Source: CAD feature listing. Evaluate the final solid. Frame: model axes, mm. A direction names the side the tool comes from. Round coordinates to 2 decimals unless told otherwise and drop trailing zeros. Write each loop counter-clockwise with the first axis right and the second up, starting at its lowest first coordinate (ties: lowest second). Pieces come first, ordered by that corner, then holes. Notation, with made-up numbers: M -2.5,50.5 L 38.5,50.5 A37 ccw 38.5,88.5 Z; hole C -15.75,47 d9. An arc over 180 degrees is marked long. Answer in a Markdown table with one row per item.
from build123d import *

# Parameters (mm, degrees)
SKETCH2_R           = 17.6
BOSS_EXTRUDE1_DEPTH = 52.5
SKETCH3_R           = 2.1
BOSS_EXTRUDE2_DEPTH = 7.6
SKETCH4_W           = 1.23
SKETCH4_H           = 14.7
BOSS_EXTRUDE3_DEPTH = 3.5
CUT_EXTRUDE1_START  = -3
SKETCH5_R           = 17.6
SKETCH5_R_2         = 4.5
SKETCH5_W           = 1.23
SKETCH5_H           = 14.7
SKETCH5_R_3         = 2.5
CUT_EXTRUDE1_DEPTH  = 3
SKETCH7_R           = 19.95
BOSS_EXTRUDE5_DEPTH = 5.5
FILLET3_R           = 5
FILLET4_R           = 0.5
CUT_EXTRUDE2_START  = -7
SKETCH8_R           = 2.5
CUT_EXTRUDE2_DEPTH  = 7
SKETCH10_R          = 2.8
BOSS_EXTRUDE6_DEPTH = 8.6
FILLET5_R           = 0.5


with BuildPart() as part:
    # Sketch2 → Boss-Extrude1 (new body)
    with BuildSketch(Plane.XY):
        Circle(SKETCH2_R)
    extrude(amount=BOSS_EXTRUDE1_DEPTH)

    # Sketch3 → Boss-Extrude2 (add)
    # profile 1 of 2: a face of its own
    with BuildSketch(Plane.XY):
        with BuildLine():
            Line((-10.476190476, 14.14246913), (-25.391666667, 3.093665122))
            ThreePointArc((-25.391666667, 3.093665122), (-26.95, 0), (-25.391666667, -3.093665122))
            Line((-25.391666667, -3.093665122), (-10.476190476, -14.14246913))
            ThreePointArc((-10.476190476, -14.14246913), (-17.6, 0), (-10.476190476, 14.14246913))
        make_face()
        with Locations(Location((-23.1, 0, 0), (0, 0, 180))):
            Circle(SKETCH3_R, mode=Mode.SUBTRACT)
    # profile 2 of 2: a face of its own
    with BuildSketch(Plane.XY):
        with BuildLine():
            Line((25.391666667, 3.093665122), (10.476190476, 14.14246913))
            ThreePointArc((10.476190476, 14.14246913), (17.6, 0), (10.476190476, -14.14246913))
            Line((10.476190476, -14.14246913), (25.391666667, -3.093665122))
            ThreePointArc((25.391666667, -3.093665122), (26.95, 0), (25.391666667, 3.093665122))
        make_face()
        with Locations(Location((23.1, 0, 0), (0, 0, 180))):
            Circle(SKETCH3_R, mode=Mode.SUBTRACT)
    extrude(amount=BOSS_EXTRUDE2_DEPTH)

    # Sketch4 → Boss-Extrude3 (add)
    with BuildSketch(Plane.XY.offset(52.5)):
        Rectangle(SKETCH4_W, SKETCH4_H)
    extrude(amount=BOSS_EXTRUDE3_DEPTH)

    # Sketch5 → Cut-Extrude1 (cut)
    # profile 1 of 3: a face of its own
    with BuildSketch(Plane.XY.offset(52.5).offset(CUT_EXTRUDE1_START)):
        with Locations(Location((0, 0, 0), (0, 0, 126.52960723))):
            Circle(SKETCH5_R)
        with Locations((-8.9, 0)):
            Circle(SKETCH5_R_2, mode=Mode.SUBTRACT)
        with Locations((8.9, 0)):
            Circle(SKETCH5_R_2, mode=Mode.SUBTRACT)
        Rectangle(SKETCH5_W, SKETCH5_H, mode=Mode.SUBTRACT)
    # profile 2 of 3: a face of its own
    with BuildSketch(Plane.XY.offset(52.5).offset(CUT_EXTRUDE1_START)):
        with Locations((-8.9, 0)):
            Circle(SKETCH5_R_3)
    # profile 3 of 3: a face of its own
    with BuildSketch(Plane.XY.offset(52.5).offset(CUT_EXTRUDE1_START)):
        with Locations((8.9, 0)):
            Circle(SKETCH5_R_3)
    extrude(amount=CUT_EXTRUDE1_DEPTH, mode=Mode.SUBTRACT)

    # Sketch7 → Boss-Extrude5 (add)
    with BuildSketch(Plane.XY.offset(49.5)):
        Circle(SKETCH7_R)
    extrude(amount=-BOSS_EXTRUDE5_DEPTH)

    # Fillet3
    # the kernel refuses this fillet: 5 mm, written as the material it adds along each edge
    with BuildSketch(Plane(origin=(0, 0, 44), x_dir=(1, 0, 0), z_dir=(0, 1, 0))) as fillet3_piece_1:
        with BuildLine():
            CenterArc((22.6, 4.239988208), FILLET3_R, 180, 57.994545172)
            Line((19.95, 0), (19.897, -0.084799764))
            ThreePointArc((19.897, -0.084799764), (18.775, -0.1), (17.6, -0.1))
            Line((17.6, -0.1), (17.5, 0))
            Line((17.5, 0), (17.5, 4.239988208))
            Line((17.5, 4.239988208), (17.6, 4.239988208))
        make_face()
    revolve(axis=Axis((0, 0, 44), (0, 0, -1)))

    # Fillet4
    fillet4_edges = [part.edges().sort_by_distance(p)[0] for p in [
        (0.615, 0, 56),
        (0, 7.35, 56),
        (0, -7.35, 56),
        (-0.615, 0, 56),
        (0, 7.35, 49.5),
        (-0.615, 0, 49.5),
        (0, -7.35, 49.5),
        (0.615, 0, 49.5),
        (-13.4, 0, 49.5),
        (4.4, 0, 49.5),
        (-19.95, 0, 49.5),
    ]]
    fillet(fillet4_edges, radius=FILLET4_R)

    # Sketch8 → Cut-Extrude2 (cut)
    with BuildSketch(Plane.XY.offset(52.5).offset(CUT_EXTRUDE2_START)):
        with Locations((8.9, 0)):
            Circle(SKETCH8_R)
        with Locations((-8.9, 0)):
            Circle(SKETCH8_R)
    extrude(amount=CUT_EXTRUDE2_DEPTH, mode=Mode.SUBTRACT)

    # Sketch10 → Boss-Extrude6 (add)
    with BuildSketch(Plane.XY.offset(49.5)):
        with Locations(Location((0, 12.15, 0), (0, 0, 180))):
            Circle(SKETCH10_R)
    extrude(amount=BOSS_EXTRUDE6_DEPTH)

    # Fillet5
    fillet5_edges = [part.edges().sort_by_distance(p)[0] for p in [
        (2.8, 12.15, 58.1),
    ]]
    fillet(fillet5_edges, radius=FILLET5_R)


solid = part.part
Q1. Contact query for flat-ended pins moving along their axis: pin 1 Ø4 at (x, z) = (15, 16.5) entering from +Y; pin 2 Ø4.5 at (y, z) = (-2, 51.5) entering from -X; pin 3 Ø1 at (x, z) = (-14, 21) entering from -Y. Output: stop coordinate, or through.
Solutions:
| item | result |
|---|---|
| pin 1 | stops at y = 11.86 |
| pin 2 | stops at x = -19.8 |
| pin 3 | stops at y = -11.29 |
Q2. Material intervals for probe 1 along X at (y, z) = (0.5, 51) (3 decimals); probe 2 along Y at (x, z) = (-8.9, 51); probe 3 along Z at (x, y) = (-12, -6), sorted ascending.
Solutions:
| item | result |
|---|---|
| probe 1 | x = -13.372 to -11.349, -6.451 to -4.428, -0.615 to 0.615, 4.428 to 6.451, 11.349 to 13.372 |
| probe 2 | y = -4.5 to -2.5, 2.5 to 4.5 |
| probe 3 | z = 0 to 49.5 |
Q3. Access query for faces 4 (the flat face through (-7, -2, 52.5)), 5 (the flat face through (17.83, -8.695, 3.747)), 6 (the flat face through (4, -4, 49.5)), 7 (the flat face through (11, -2, 52.5)). Directions: +Z, -Z, +X, -X, +Y, -Y. A direction counts if a zero-diameter tool reaches every point of the face in a straight line with its end or side. Return the directions, or none.
Solutions:
| item | result |
|---|---|
| face 4 | +Z, -X, +Y, -Y |
| face 5 | -Z, +X, -Y |
| face 6 | +Z |
| face 7 | +Z, +X, +Y, -Y |
Q4. Section A-A (z = 27.5). Return loops of the section in (x, y), and give its area (3 significant figures).
Solutions:
| item | result |
|---|---|
| outline | C 0,0 d35.2 |
| area | 973 mm2 |
Q5. Pull-direction query (Y, two-part tool) for faces 1 (the flat face through (-0.615, 0, 53)), 2 (the cylindrical face through (-13.396, 0.198, 51.232)), 3 (the cylindrical face through (21.097, -0.631, 3.747)); classes: pulls with the +Y half, pulls with the -Y half, needs draft (parallel to the pull), parting line crosses it, or undercut.
Solutions:
| item | result |
|---|---|
| face 1 | needs draft |
| face 2 | parting line crosses it |
| face 3 | undercut |
